Autodesk Inventor part; units mm, degrees
ref_plane "Start Plane" through (0, 10, 0) normal (0, 1, 0) x (-1, 0, 0)
ref_plane "End Plane" through (0, 294.8, 0) normal (0, 1, 0) x (-1, 0, 0)
ref_plane "Work Plane5" through (0, 294.8, 3.5) normal (0, 1, 0) x (1, 0, 0)
ref_plane "Start Plane" through (0, 10, 0) normal (0, 1, 0) x (-1, 0, 0)
ref_plane "End Plane" through (0, 294.8, 0) normal (0, 1, 0) x (-1, 0, 0)
sketch "Sketch" plane through (0, 0, 0) normal (0, 1, 0) x (-1, 0, 0)
  line L0 (-1.7574, 4) -> (1.7574, 4)
  line L1 (4, 1.7574) -> (4, -1.7574)
  line L2 (1.7574, -4) -> (-1.7574, -4)
  line L3 (-4, -1.7574) -> (-4, 1.7574)
  line L4 (4.5858, -3.1716) -> (7.1464, -5.7322)
  line L5 (3.1716, -4.5858) -> (5.7322, -7.1464)
  line L6 (5.3787, -8) -> (3.5, -8)
  line L7 (3, -8.5) -> (3, -9.5)
  line L8 (3.5, -10) -> (9, -10)
  line L9 (10, -9) -> (10, -3.5)
  line L10 (9.5, -3) -> (8.5, -3)
  line L11 (8, -3.5) -> (8, -5.3787)
  line L12 (4, 0) -> (-4, 0) construction
  line L13 (0, -4) -> (0, 4) construction
  arc A0 (4, -1.7574) -> (4.5858, -3.1716) centre (6, -1.7574) ccw
  arc A1 (3.1716, -4.5858) -> (1.7574, -4) centre (1.7574, -6) ccw
  arc A2 (3.5, -8) -> (3, -8.5) centre (3.5, -8.5) ccw
  arc A3 (3, -9.5) -> (3.5, -10) centre (3.5, -9.5) ccw
  arc A4 (10, -3.5) -> (9.5, -3) centre (9.5, -3.5) ccw
  arc A5 (8.5, -3) -> (8, -3.5) centre (8.5, -3.5) ccw
  arc A6 (7.1464, -5.7322) -> (8, -5.3787) centre (7.5, -5.3787) ccw
  arc A7 (5.3787, -8) -> (5.7322, -7.1464) centre (5.3787, -7.5) ccw
  arc A8 (9, -10) -> (10, -9) centre (9, -9) ccw
  line L14 (-4.5858, -3.1716) -> (-7.1464, -5.7322)
  line L15 (-3.1716, -4.5858) -> (-5.7322, -7.1464)
  line L16 (-5.3787, -8) -> (-3.5, -8)
  line L17 (-3, -8.5) -> (-3, -9.5)
  line L18 (-3.5, -10) -> (-9, -10)
  line L19 (-10, -9) -> (-10, -3.5)
  line L20 (-9.5, -3) -> (-8.5, -3)
  line L21 (-8, -3.5) -> (-8, -5.3787)
  arc A9 (-4.5858, -3.1716) -> (-4, -1.7574) centre (-6, -1.7574) ccw
  arc A10 (-1.7574, -4) -> (-3.1716, -4.5858) centre (-1.7574, -6) ccw
  arc A11 (-3, -8.5) -> (-3.5, -8) centre (-3.5, -8.5) ccw
  arc A12 (-3.5, -10) -> (-3, -9.5) centre (-3.5, -9.5) ccw
  arc A13 (-9.5, -3) -> (-10, -3.5) centre (-9.5, -3.5) ccw
  arc A14 (-8, -3.5) -> (-8.5, -3) centre (-8.5, -3.5) ccw
  arc A15 (-8, -5.3787) -> (-7.1464, -5.7322) centre (-7.5, -5.3787) ccw
  arc A16 (-5.7322, -7.1464) -> (-5.3787, -8) centre (-5.3787, -7.5) ccw
  arc A17 (-10, -9) -> (-9, -10) centre (-9, -9) ccw
  line L22 (4.5858, 3.1716) -> (7.1464, 5.7322)
  line L23 (3.1716, 4.5858) -> (5.7322, 7.1464)
  line L24 (5.3787, 8) -> (3.5, 8)
  line L25 (3, 8.5) -> (3, 9.5)
  line L26 (3.5, 10) -> (9, 10)
  line L27 (10, 9) -> (10, 3.5)
  line L28 (9.5, 3) -> (8.5, 3)
  line L29 (8, 3.5) -> (8, 5.3787)
  arc A18 (4.5858, 3.1716) -> (4, 1.7574) centre (6, 1.7574) ccw
  arc A19 (1.7574, 4) -> (3.1716, 4.5858) centre (1.7574, 6) ccw
  arc A20 (3, 8.5) -> (3.5, 8) centre (3.5, 8.5) ccw
  arc A21 (3.5, 10) -> (3, 9.5) centre (3.5, 9.5) ccw
  arc A22 (9.5, 3) -> (10, 3.5) centre (9.5, 3.5) ccw
  arc A23 (8, 3.5) -> (8.5, 3) centre (8.5, 3.5) ccw
  arc A24 (8, 5.3787) -> (7.1464, 5.7322) centre (7.5, 5.3787) ccw
  arc A25 (5.7322, 7.1464) -> (5.3787, 8) centre (5.3787, 7.5) ccw
  arc A26 (10, 9) -> (9, 10) centre (9, 9) ccw
  line L30 (-10, 9) -> (-10, 3.5)
  arc A27 (-9, 10) -> (-10, 9) centre (-9, 9) ccw
  arc A28 (-10, 3.5) -> (-9.5, 3) centre (-9.5, 3.5) ccw
  line L31 (-9.5, 3) -> (-8.5, 3)
  arc A29 (-8.5, 3) -> (-8, 3.5) centre (-8.5, 3.5) ccw
  line L32 (-8, 3.5) -> (-8, 5.3787)
  arc A30 (-7.1464, 5.7322) -> (-8, 5.3787) centre (-7.5, 5.3787) ccw
  line L33 (-4.5858, 3.1716) -> (-7.1464, 5.7322)
  line L34 (-3.1716, 4.5858) -> (-5.7322, 7.1464)
  arc A31 (-3.1716, 4.5858) -> (-1.7574, 4) centre (-1.7574, 6) ccw
  arc A32 (-4, 1.7574) -> (-4.5858, 3.1716) centre (-6, 1.7574) ccw
  arc A33 (-5.3787, 8) -> (-5.7322, 7.1464) centre (-5.3787, 7.5) ccw
  line L35 (-5.3787, 8) -> (-3.5, 8)
  arc A34 (-3.5, 8) -> (-3, 8.5) centre (-3.5, 8.5) ccw
  line L36 (-3, 8.5) -> (-3, 9.5)
  arc A35 (-3, 9.5) -> (-3.5, 10) centre (-3.5, 9.5) ccw
  line L37 (-3.5, 10) -> (-9, 10)
  circle A36 centre (0, 0) radius 2.5
  point P0 (3, -8)
  point P1 (3, -10)
  point P2 (10, -10)
  dimension "d3" = 2
  dimension "d4" = 2
  dimension "d5" = 7
  dimension "d6" = 2
  dimension "d7" = 0.5
  dimension "d8" = 1
  dimension "d9" = 20
  dimension "d10" = 20
  dimension "d11" = 8
  dimension "d13" = 5
  dimension "d14" = 8
extrude "Body" add sketch "Sketch" along normal up to surface (284.8 mm away) from surface at 10
sketch "Sketch4" plane through (0, 0, 0) normal (0, 1, 0) x (-1, 0, 0)
  line L0 (0, 0) -> (10, 0)
ref_plane "Work Plane4" through (0, 0, 0) normal (0, 0, -1) x (-1, 0, 0)
sketch "Sketch5" plane through (0, 0, 0) normal (0, 0, -1) x (-1, 0, 0)
  line L0 (-2, 10) -> (12, 10)
  line L1 (-2, 294.8) -> (12, 294.8)
  dimension "d22" = 284.8
ref_plane "Work Plane5" through (0, 294.8, 3.5) normal (0, 1, 0) x (1, 0, 0)
split "Split1" plane through (0, 294.8, 3.5) removes the side toward (0, 1, 0)
ref_plane "Work Plane6" through (-279.4, 10, 3.5) normal (0, -1, 0) x (1, 0, 0)
split "Split2" plane through (-279.4, 10, 3.5) removes the side toward (0, -1, 0)
equation "\"d18\" = Length + G_OFFSET_END"
equation "\"G_L\" = d22"
properties part number "A3.3"
Can you work these out from the model? Positions are in its coordinate system, mm. Round coordinates to 2 decimals unless told otherwise and drop trailing zeros.
Item 1: Please list where these lines run through material, in increasing order: L1, parallel to Z at x = -7.5, y = 88.5; L2, parallel to Z at x = 0, y = 187; L3, parallel to X at y = 211, z = -5.
Item 2: Will these pins go through, and if not, where does the flat tip stop? pin 1 Ø1 at (y, z) = (42.5, -1) entering from +X; pin 2 Ø3 at (y, z) = (89.5, -1) entering from +X; pin 3 Ø1.5 at (x, y) = (2.5, 258.5) entering from +Z.
Item 3: If we mould it in two halves opening along Z, with no side actions, what happens to faces 1 (the flat face through (10, 150, 6)), 2 (the flat face through (-6, 150, 10)), 3 (the cylindrical face through (0.54, 150.41, 2.44))? For each: +Z half, -Z half, draft (parallel to the pull), parting line (faces both ways), or undercut.
Reported:
1. L1: z = -10 to -5.88, 5.88 to 10
1. L2: z = -4 to -2.5, 2.5 to 4
1. L3: x = -10 to -8, -6.41 to -3.59, 3.59 to 6.41, 8 to 10
2. pin 1: stops at x = 4
2. pin 2: stops at x = 4.14
2. pin 3: stops at z = 9.93
3. face 1: draft
3. face 2: +Z half
3. face 3: undercut
